```python
from build123d import *

# Parameters (mm, degrees)
F0_W     = 200
F0_H     = 100
F0_R     = 35
F1_DEPTH = 25
F2_W     = 9.490147
F2_H     = 100
F2_W_2   = 17.155282
F3_DEPTH = 10


with BuildPart() as f1:
    # F0 (on Top) → F1 (new body)
    with BuildSketch(Plane.XY):
        Rectangle(F0_W, F0_H)
        Circle(F0_R, mode=Mode.SUBTRACT)
    extrude(amount=F1_DEPTH)

    # F2 (on face) → F3 (cut)
    with BuildSketch(Plane.XY.offset(25)):
        with Locations((-78.019992, 0)):
            Rectangle(F2_W, F2_H)
        with Locations((73.092412, 0)):
            Rectangle(F2_W_2, F2_H)
    extrude(amount=-F3_DEPTH, mode=Mode.SUBTRACT)


solid = f1.part
```
Work out the finished part from the listing and answer in its coordinate system (mm). A direction names the side the tool comes from. Give positions to 0.01 mm unless a question says otherwise; leave off trailing zeros. Order: outer loops, then holes, each group sorted by start corner. A loop starts at its lowest first (then second) coordinate and runs counter-clockwise, first axis right, second up. Notation, with made-up numbers: M 41,15 L 61,15 A13 cw 61,33 Z; hole C -24.5,-33 d10. An arc over 180 degrees is marked long. Return JSON: item names as keys, results as strings.
1) Section C-C, the plane y = 27 is taken. Write down the section's boundary in (x, z).
Resolved:
{"outline": "M -100,0 L -22.27,0 L -22.27,25 L -73.27,25 L -73.27,15 L -82.77,15 L -82.77,25 L -100,25 Z; M 22.27,0 L 100,0 L 100,25 L 81.67,25 L 81.67,15 L 64.51,15 L 64.51,25 L 22.27,25 Z"}
2) A tool of negligible diameter and unlimited length cuts with its end or side. For faces 4 (the flat face through (91, 1, 25)), 5 (the flat face through (64.515, -1, 20)), from which of +Z, -Z, +X, -X, +Y, -Y can it reach the whole face along a straight path? Write none if from no direction.
Resolved:
{"face 4": "+Z, +X, -X, +Y, -Y", "face 5": "+Z, +Y, -Y"}
3) Section B-B, the plane y = 0 is taken. Write down the section's boundary in (x, z), plus the area to 3 significant figures.
Resolved:
{"outline": "M -100,0 L -35,0 L -35,25 L -73.27,25 L -73.27,15 L -82.77,15 L -82.77,25 L -100,25 Z; M 35,0 L 100,0 L 100,25 L 81.67,25 L 81.67,15 L 64.51,15 L 64.51,25 L 35,25 Z", "area": "2,980 mm^2"}
4) Section D-D, the plane x = 27.5 is taken. Write down the section's boundary in (y, z).
Resolved:
{"outline": "M -50,0 L -21.65,0 L -21.65,25 L -50,25 Z; M 21.65,0 L 50,0 L 50,25 L 21.65,25 Z"}
5) Straight lines are drawn through the part: line 1 along Y through (x, z) = (0, 11.25); line 2 along X through (y, z) = (-1, 4.5); line 3 along Z through (x, y) = (66.5, -2.5). For each, find the intervals that lie inside material, in ascending order. Write a range as [from, to].
Resolved:
{"line 1": "[-50, -35], [35, 50]", "line 2": "[-100, -34.99], [34.99, 100]", "line 3": "[0, 15]"}
6) Each of these flat-tipped pins is pushed along its axis until it touches: pin 1 (3 mm diameter, centred on x = -79, y = 24.5, fed in from +Z); pin 2 (3 mm diameter, centred on x = -27.5, y = -20.5, fed in from +Z). Where does it stop, or does it pass through?
Resolved:
{"pin 1": "z = 15", "pin 2": "z = 25"}
7) For a pull along X with two mould halves and no side action, classify faces 1 (the cylindrical face through (-28, -21, 12)), 2 (the flat face through (100, -1, 12)), 3 (the flat face through (-36, 1, 25)) as +X half, -X half, draft (parallel to the pull), parting line (faces both ways), or undercut.
Resolved:
{"face 1": "undercut", "face 2": "+X half", "face 3": "draft"}
8) Section A-A, the plane x = 0 is taken. Write down the section's boundary in (y, z), plus the area to 3 significant figures.
Resolved:
{"outline": "M -50,0 L -35,0 L -35,25 L -50,25 Z; M 35,0 L 50,0 L 50,25 L 35,25 Z", "area": "750 mm^2"}
